from build123d import *

# Parameters (mm, degrees)
SKETCH004_W      = 2
SKETCH004_H      = 4.6
EXTRUDE004_DEPTH = 4.6
SKETCH003_W      = 4
SKETCH003_H      = 6.2
EXTRUDE003_DEPTH = 3.4
EXTRUDE002_DEPTH = 10.2
EXTRUDE001_DEPTH = 10.4
SKETCH005_W      = 2.2
SKETCH005_H      = 2.2
EXTRUDE005_DEPTH = 12.6
SKETCH006_W      = 2.2
SKETCH006_H      = 2.2
EXTRUDE006_DEPTH = 12.6
SKETCH_W         = 4
SKETCH_H         = 50
EXTRUDE_DEPTH    = 12.6


with BuildPart() as extrude004_led:
    # Sketch004 → Extrude004 (new body, symmetric)
    with BuildSketch(Plane.XZ):
        with Locations((1, 5.3)):
            Rectangle(SKETCH004_W, SKETCH004_H)
    extrude(amount=EXTRUDE004_DEPTH, both=True)


with BuildPart() as obj1:
    # Sketch003 → Extrude003 (new body, symmetric)
    with BuildSketch(Plane.XZ):
        with Locations((2, 13.1)):
            Rectangle(SKETCH003_W, SKETCH003_H)
    extrude(amount=EXTRUDE003_DEPTH, both=True)


with BuildPart() as extrude002_step_down:
    # Sketch002 → Extrude002 (new body, symmetric)
    with BuildSketch(Plane.XZ):
        Polygon((0, 18), (2.6, 18), (2.6, 29.4), (0, 29.4), (-3.8, 29.4), (-3.8, 18), align=None)
    extrude(amount=EXTRUDE002_DEPTH, both=True)


with BuildPart() as extrude001_power_path:
    # Sketch001 → Extrude001 (new body, symmetric)
    with BuildSketch(Plane.XZ):
        Polygon((0, 30.4), (3, 30.4), (3, 46), (0, 46), (-3.8, 46), (-3.8, 30.4), align=None)
    extrude(amount=EXTRUDE001_DEPTH, both=True)


with BuildPart() as obj2:
    # Sketch005 → Extrude005 (new body, symmetric)
    with BuildSketch(Plane.XZ):
        with BuildLine():
            Line((-3.8, 43.6), (-3.8, 41.4))
            ThreePointArc((-3.8, 41.4), (-3.331371, 40.268629), (-2.2, 39.8))
            Line((-2.2, 39.8), (1.6, 39.8))
            Line((1.6, 39.8), (1.6, 45.2))
            Line((1.6, 45.2), (-2.2, 45.2))
            ThreePointArc((-2.2, 45.2), (-3.331371, 44.731371), (-3.8, 43.6))
        make_face()
        with Locations((-1.1, 42.5)):
            Rectangle(SKETCH005_W, SKETCH005_H, mode=Mode.SUBTRACT)
    extrude(amount=EXTRUDE005_DEPTH, both=True)


with BuildPart() as obj3:
    # Sketch006 → Extrude006 (new body, symmetric)
    with BuildSketch(Plane.XZ):
        with BuildLine():
            Line((-3.8, 27.4), (-3.8, 25.2))
            ThreePointArc((-3.8, 25.2), (-3.331371, 24.068629), (-2.2, 23.6))
            Line((-2.2, 23.6), (1.6, 23.6))
            Line((1.6, 23.6), (1.6, 29))
            Line((1.6, 29), (-2.2, 29))
            ThreePointArc((-2.2, 29), (-3.331371, 28.531371), (-3.8, 27.4))
        make_face()
        with Locations((-1.1, 26.3)):
            Rectangle(SKETCH006_W, SKETCH006_H, mode=Mode.SUBTRACT)
    extrude(amount=EXTRUDE006_DEPTH, both=True)


with BuildPart() as cut003:
    # Sketch → Extrude (new body, symmetric)
    with BuildSketch(Plane.XZ):
        with Locations((2, 25)):
            Rectangle(SKETCH_W, SKETCH_H)
    extrude(amount=EXTRUDE_DEPTH, both=True)

    # Fusion: union obj2, obj3
    add(obj2.part)
    add(obj3.part)

    # Cut: cut Extrude001 - power - path
    add(extrude001_power_path.part, mode=Mode.SUBTRACT)

    # Cut001: cut Extrude002 - step -down
    add(extrude002_step_down.part, mode=Mode.SUBTRACT)

    # Cut002: cut obj1
    add(obj1.part, mode=Mode.SUBTRACT)

    # Cut003: cut Extrude004 - led
    add(extrude004_led.part, mode=Mode.SUBTRACT)


solid = cut003.part
The model under review builds one solid part; all positions refer to its coordinate system, in mm. A direction names the side the tool comes from. Round coordinates to 2 decimals unless told otherwise and drop trailing zeros. Order: outer loops, then holes, each group sorted by start corner. A loop starts at its lowest first (then second) coordinate and runs counter-clockwise, first axis right, second up. Notation, with made-up numbers: (54, -40) -> (101, -40) arc R28 cw to (101, -20) -> close; hole circle Ø9 at (35, 48). An arc over 180 degrees is marked (long way). Use CSV: the item, a comma, the result in double quotes. Start each with the question number.
(1) Consider section B-B on x = 3.5. Write out the cut boundary in (y, z).
(2) Insertion check: pin 1 (0.7 mm diameter, centred on x = -0.5, y = -12, fed in from +Z); pin 2 (2.5 mm diameter, centred on x = -1.5, y = 11, fed in from -Z); pin 3 (3 mm diameter, centred on y = 4.5, z = 34.5, fed in from -X). Each pin has a flat end and moves straight along its axis. Give the tip position at first contact, or say it passes through.
(3) Consider section A-A on z = 11.5. Write out the cut boundary in (x, y), and give its area (3 significant figures).
(4) Consider section D-D on x = -0.75. State how many separate pieces and enclosed holes the cut face has, and give its area (3 significant figures).
(5) Wall thickness on probe 1 along Z at (x, y) = (1.5, -9.25); probe 2 along Z at (x, y) = (-1.5, -11); probe 3 along Y at (x, z) = (0, 40.5): over which ranges is each line inside the solid? List them lowest first. Write a range as from..to.
(6) Tool access review of faces 4 (the face through (-1, 11, 29)), 5 (the face through (-1, -12, 45.2)), 6 (the face through (1, 0, 3)), 7 (the face through (-2.2, -11, 26)), 8 (the face through (0, 0, 9)): name each direction out of +Z, -Z, +X, -X, +Y, -Y from which nothing blocks a thin tool from reaching the whole face with its end or side.
(7) Mouldability with a two-part tool opening along X and no side actions: class faces 1 (the face through (-1, 11, 39.8)), 2 (the face through (-3.34, -11.52, 40.28)), 3 (the face through (-1, -11, 25.2)) as pulls with the +X half, pulls with the -X half, needs draft (parallel to the pull), parting line crosses it, or undercut.
(8) Consider section C-C on y = 0.5. Write out the cut boundary in (x, z), and give its area (3 significant figures).
Responses:
1,outline,"(-12.6, 0) -> (12.6, 0) -> (12.6, 50) -> (-12.6, 50) -> close; hole (-3.4, 10) -> (3.4, 10) -> (3.4, 16.2) -> (-3.4, 16.2) -> close"
2,pin 1,"z = 45.2"
2,pin 2,"z = 23.6"
2,pin 3,"x = 3"
3,outline,"(0, -12.6) -> (4, -12.6) -> (4, -3.4) -> (0, -3.4) -> close; (0, 3.4) -> (4, 3.4) -> (4, 12.6) -> (0, 12.6) -> close"
3,area,"73.6 mm²"
4,separate pieces,"8"
4,enclosed holes,"0"
4,area,"29.4 mm²"
5,probe 1,"0..18, 29.4..30.4, 46..50"
5,probe 2,"23.6..25.2, 27.4..29, 39.8..41.4, 43.6..45.2"
5,probe 3,"-12.6..-10.4, 10.4..12.6"
6,face 4,"-X, +Y, -Y"
6,face 5,"+Z, -X, +Y, -Y"
6,face 6,"-X"
6,face 7,"+Y, -Y"
6,face 8,"-Z, -X, +Y, -Y"
7,face 1,"needs draft"
7,face 2,"pulls with the -X half"
7,face 3,"undercut"
8,outline,"(0, 0) -> (4, 0) -> (4, 10) -> (0, 10) -> (0, 7.6) -> (2, 7.6) -> (2, 3) -> (0, 3) -> close; (0, 16.2) -> (4, 16.2) -> (4, 50) -> (0, 50) -> (0, 46) -> (3, 46) -> (3, 30.4) -> (0, 30.4) -> (0, 29.4) -> (2.6, 29.4) -> (2.6, 18) -> (0, 18) -> close"
8,area,"89.6 mm²"
